Verification items for this drawing (mm, ordinates from the low corner). A direction names the side the tool comes from. Give positions to 0.01 mm unless a question says otherwise; leave off trailing zeros. Loops run counter-clockwise (first coordinate to the right, second up) from the corner with the lowest first, then second, coordinate; pieces in that order, holes last. Notation, with made-up numbers: M 14,-22.5 L 43,-22.5 A15 cw 43,-4.5 Z; hole C 75,73.5 d4. An arc over 180 degrees is marked long. Answer in a Markdown table with one row per item.
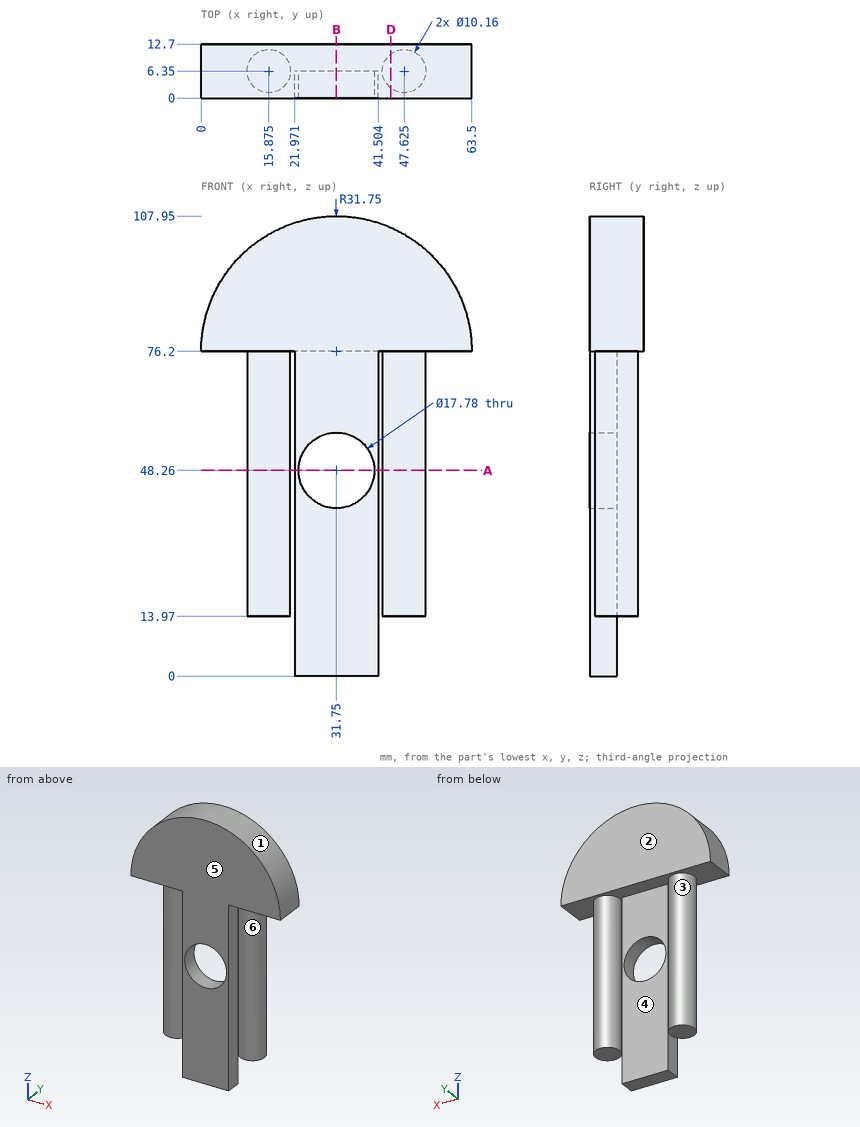
Item 1: Release check for a two-part mould opening along X. For the marked faces 1, 2 and 3 record: released by +X, released by -X, zero draft, split by the parting line, or undercut.
Reported:
| item | result |
|---|---|
| face 1 | split by the parting line |
| face 2 | zero draft |
| face 3 | undercut |
Item 2: Sectioned sample at A-A (z = 48.26). State how many separate pieces and enclosed holes the cut face has, and give its area (3 significant figures).
Reported:
| item | result |
|---|---|
| separate pieces | 4 |
| enclosed holes | 0 |
| area | 173 mm^2 |
Item 3: Tool access check on the marked faces 4, 5 and 6. Record the directions out of +Z, -Z, +X, -X, +Y, -Y that give a thin tool (end or side, any length) a straight path to the whole face; none if there is none.
Reported:
| item | result |
|---|---|
| face 4 | -Z, +Y |
| face 5 | +Z, -Z, +X, -X, -Y |
| face 6 | -Z |
Item 4: Scan lines: L1, parallel to X at y = 5.5, z = 32.5; L2, parallel to X at y = 4.5, z = 64 (1 decimal); L3, parallel to Y at x = 47.5, z = 72. Record each from-to range of solid material in increasing order. Write a range as [from, to].
Reported:
| item | result |
|---|---|
| L1 | x = [10.87, 20.88], [21.97, 41.5], [42.62, 52.63] |
| L2 | x = [11.1, 20.6], [22, 41.5], [42.9, 52.4] |
| L3 | y = [1.27, 11.43] |
Item 5: Go/stop test with flat-tipped pins: pin 1 (1.5 mm diameter, centred on x = 55, y = 5, fed in from -Z); pin 2 (8 mm diameter, centred on x = 46.5, z = 22.5, fed in from +Y); pin 3 (3 mm diameter, centred on y = 2.5, z = 45.5, fed in from +X). Record where each tip stops, or that it passes through.
Reported:
| item | result |
|---|---|
| pin 1 | stops at z = 76.2 |
| pin 2 | stops at y = 11.43 |
| pin 3 | stops at x = 52.13 |
Item 6: Sectioned sample at D-D (x = 44.5). Record the cut outline in (y, z) (1 decimal).
Reported:
| item | result |
|---|---|
| outline | M 0,76.2 L 2.3,76.2 L 2.3,14 L 10.4,14 L 10.4,76.2 L 12.7,76.2 L 12.7,105.3 L 0,105.3 Z |
Item 7: Sectioned sample at B-B (x = 31.75). Record the cut outline in (y, z).
Reported:
| item | result |
|---|---|
| outline | M 0,0 L 6.35,0 L 6.35,39.37 L 0,39.37 Z; M 0,57.15 L 6.35,57.15 L 6.35,76.2 L 12.7,76.2 L 12.7,107.95 L 0,107.95 Z |
